Drawing for the job (mm, zero at the part's lowest x, y, z). A direction names the side the tool comes from. Round coordinates to 2 decimals unless told otherwise and drop trailing zeros. Order: outer loops, then holes, each group sorted by start corner. A loop starts at its lowest first (then second) coordinate and runs counter-clockwise, first axis right, second up. Notation, with made-up numbers: (63, 49.25) - (77, 49.25) arc R29 cw to (77, 71.25) - close; hole circle Ø11 at (10, 59). An arc over 180 degrees is marked (long way). Put each result on its own line as item: value. Start each with the question number.
Item 1: Mould opens along Z. For the marked faces 1, 2 and 3 say: pulls with the +Z half, pulls with the -Z half, needs draft (parallel to the pull), parting line crosses it, or undercut.
Item 2: Saw through at D-D on z = 20.25. List the corners of the cut face in (x, y) (3 decimals).
Item 3: Pin check, flat tip, straight feed: pin 1 Ø5.5 at (y, z) = (50.8, 12.7) entering from -X. Stop position of the tip, or through.
Item 4: Saw through at A-A on y = 139.7. List the corners of the cut face in (x, z) (3 decimals).
Item 5: Saw through at C-C on z = 12.7. List the corners of the cut face in (x, y) (3 decimals), plus the area to 3 significant figures.
Item 6: Probe probe 1 along Y at (x, z) = (22.95, 12.7) (3 decimals); probe 2 along Y at (x, z) = (12.7, 0.65) (3 decimals); probe 3 along X at (y, z) = (82.5, 4.75) (3 decimals). List the from-to ranges inside material, lowest first.
Item 7: Saw through at B-B on x = 12.7. List the corners of the cut face in (y, z) (3 decimals).
Item 8: Which spindle directions (+Z, -Z, +X, -X, +Y, -Y) get a long thin tool onto all of the face, cutting with end or side? Do the marked faces 4 and 5. Say none if no direction does.
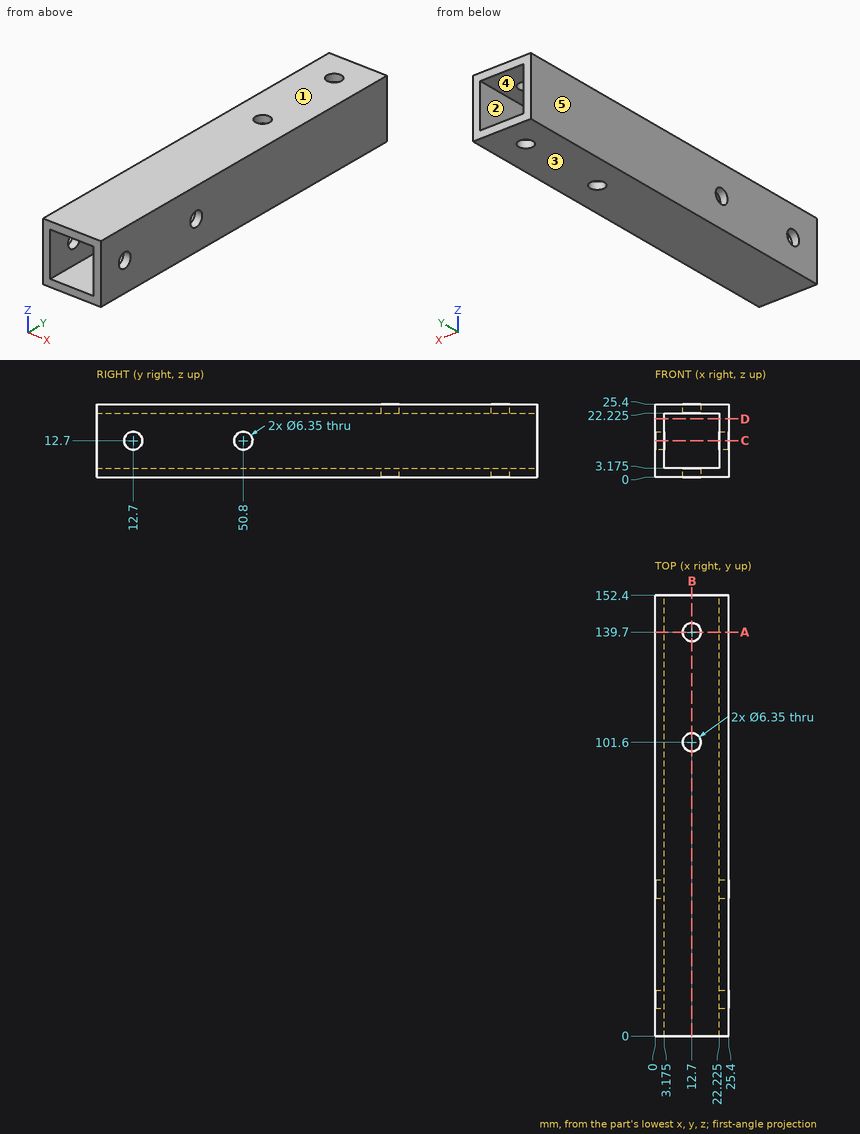
Results found:
1. face 1: pulls with the +Z half
1. face 2: undercut
1. face 3: pulls with the -Z half
2. outline: (0, 0) - (3.175, 0) - (3.175, 152.4) - (0, 152.4) - close; (22.225, 0) - (25.4, 0) - (25.4, 152.4) - (22.225, 152.4) - close
3. pin 1: passes through
4. outline: (0, 0) - (9.525, 0) - (9.525, 3.175) - (3.175, 3.175) - (3.175, 22.225) - (9.525, 22.225) - (9.525, 25.4) - (0, 25.4) - close; (15.875, 0) - (25.4, 0) - (25.4, 25.4) - (15.875, 25.4) - (15.875, 22.225) - (22.225, 22.225) - (22.225, 3.175) - (15.875, 3.175) - close
5. outline: (0, 0) - (3.175, 0) - (3.175, 9.525) - (0, 9.525) - close; (0, 15.875) - (3.175, 15.875) - (3.175, 47.625) - (0, 47.625) - close; (0, 53.975) - (3.175, 53.975) - (3.175, 152.4) - (0, 152.4) - close; (22.225, 0) - (25.4, 0) - (25.4, 9.525) - (22.225, 9.525) - close; (22.225, 15.875) - (25.4, 15.875) - (25.4, 47.625) - (22.225, 47.625) - close; (22.225, 53.975) - (25.4, 53.975) - (25.4, 152.4) - (22.225, 152.4) - close
5. area: 887 mm²
6. probe 1: y = 0 to 9.525, 15.875 to 47.625, 53.975 to 152.4
6. probe 2: y = 0 to 98.425, 104.775 to 136.525, 142.875 to 152.4
6. probe 3: x = 0 to 3.175, 22.225 to 25.4
7. outline: (0, 0) - (98.425, 0) - (98.425, 3.175) - (0, 3.175) - close; (0, 22.225) - (98.425, 22.225) - (98.425, 25.4) - (0, 25.4) - close; (104.775, 0) - (136.525, 0) - (136.525, 3.175) - (104.775, 3.175) - close; (104.775, 22.225) - (136.525, 22.225) - (136.525, 25.4) - (104.775, 25.4) - close; (142.875, 0) - (152.4, 0) - (152.4, 3.175) - (142.875, 3.175) - close; (142.875, 22.225) - (152.4, 22.225) - (152.4, 25.4) - (142.875, 25.4) - close
8. face 4: +Y, -Y
8. face 5: +Z, -Z, -X, +Y, -Y
